Geometry check sheet. Reference: the model listing, model coordinates, mm. A direction names the side the tool comes from. Coordinates: 2 decimals unless noted, no trailing zeros. Order: outer loops, then holes, each group sorted by start corner. A loop starts at its lowest first (then second) coordinate and runs counter-clockwise, first axis right, second up. Notation, with made-up numbers: M -9,-27 L 30,-27 A19 ccw 30,4 Z; hole C 43.5,6 d1. An arc over 180 degrees is marked long. Use CSV: the item, a comma, the result in double quotes. Start each with the question number.
```python
from build123d import *

# Parameters (mm, degrees)
SKETCH_28_R                  = 1
EXTRUDE_4469_DEPTH           = 38
CUT_EXTRUDE_4687_REACH       = 69.476
SKETCH_29_R                  = 1.65
CUT_EXTRUDE_4925_DEPTH       = 51.338851795
FILLET_9_R                   = 3
SKETCH_31_R                  = 1
CUT_EXTRUDE_5310_DEPTH       = 11
SKETCH_32_R                  = 3.5
CUT_EXTRUDE_5556_DEPTH       = 5
HOLE_WIZARD_5601_D           = 3.4
HOLE_WIZARD_5601_CSINK_D     = 6.3
HOLE_WIZARD_5601_CSINK_ANGLE = 90


with BuildPart() as part:
    # Эскиз28 → Extrude 4469 (new body)
    with BuildSketch(Plane.XY):
        Polygon((27, 0), (27, 11), (12, 11), (12, 14), (10, 14), (10, 30), (-20, 30), (-20, 14), (-27, 14), (-27, 11), (-27, 0), align=None)
        with Locations((3, 5.5)):
            Circle(SKETCH_28_R, mode=Mode.SUBTRACT)
        with Locations((-20, 5.5)):
            Circle(SKETCH_28_R, mode=Mode.SUBTRACT)
    extrude(amount=EXTRUDE_4469_DEPTH)

    # Эскиз29 → Cut-Extrude 4687 (cut, up to next)
    with BuildSketch(Plane.ZY.offset(20), mode=Mode.PRIVATE) as cut_extrude_4687_sk1:
        with Locations((6.5, 22)):
            Circle(SKETCH_29_R)
    cut_extrude_4687_tool1 = extrude(cut_extrude_4687_sk1.sketch, amount=-CUT_EXTRUDE_4687_REACH, mode=Mode.PRIVATE) & part.part
    # Эскиз29 → Cut-Extrude 4687 (cut, up to next)
    with BuildSketch(Plane.ZY.offset(20), mode=Mode.PRIVATE) as cut_extrude_4687_sk2:
        with Locations((31.5, 22)):
            Circle(SKETCH_29_R)
    cut_extrude_4687_tool2 = extrude(cut_extrude_4687_sk2.sketch, amount=-CUT_EXTRUDE_4687_REACH, mode=Mode.PRIVATE) & part.part
    add(cut_extrude_4687_tool1.solids().sort_by_distance((-20, 22, 6.5))[0], mode=Mode.SUBTRACT)
    add(cut_extrude_4687_tool2.solids().sort_by_distance((-20, 22, 31.5))[0], mode=Mode.SUBTRACT)

    # Эскиз30 → Cut-Extrude 4925 (cut, through all)
    with BuildSketch(Plane(origin=(0, 11, 0), x_dir=(1, 0, 0), z_dir=(0, 1, 0))):
        with BuildLine():
            Line((23, -13), (16, -13))
            Line((16, -13), (16, -25))
            Line((16, -25), (23, -25))
            ThreePointArc((23, -25), (25.898979486, -27.192752634), (27, -30.656854249))
            Line((27, -30.656854249), (27, -7.343145751))
            ThreePointArc((27, -7.343145751), (25.898979486, -10.807247366), (23, -13))
        make_face()
    extrude(amount=-CUT_EXTRUDE_4925_DEPTH, mode=Mode.SUBTRACT)

    # Скругление9
    # the kernel refuses this fillet: 3 mm, written as the material it takes off along each edge
    with BuildSketch(Plane(origin=(27, 11, 23.156854249), x_dir=(-1, 0, 0), z_dir=(0, 0, 1))) as fillet_9_piece_1:
        with BuildLine():
            CenterArc((FILLET_9_R, FILLET_9_R), FILLET_9_R, 180, 90)
            Line((0, FILLET_9_R), (0, 0))
            Line((0, 0), (FILLET_9_R, 0))
        make_face()
    extrude(amount=22.343145751, mode=Mode.SUBTRACT)
    with BuildSketch(Plane(origin=(27, 11, -7.5), x_dir=(0, -1, 0), z_dir=(0, 0, 1))) as fillet_9_piece_2:
        with BuildLine():
            CenterArc((FILLET_9_R, -FILLET_9_R), FILLET_9_R, 90, 90)
            Line((0, -FILLET_9_R), (0, 0))
            Line((0, 0), (FILLET_9_R, 0))
        make_face()
    extrude(amount=22.343145751, mode=Mode.SUBTRACT)

    # Эскиз31 → Cut-Extrude 5310 (cut)
    with BuildSketch(Plane(origin=(16, 0, 0), x_dir=(0, 0, -1), z_dir=(1, 0, 0))):
        with Locations(Location((-19, 5.5, 0), (0, 0, 90))):
            Circle(SKETCH_31_R)
    extrude(amount=-CUT_EXTRUDE_5310_DEPTH, mode=Mode.SUBTRACT)

    # Эскиз32 → Cut-Extrude 5556 (cut)
    with BuildSketch(Plane(origin=(0, 11, 0), x_dir=(1, 0, 0), z_dir=(0, 1, 0))):
        with Locations(Location((23, -6.5, 0), (0, 0, 180))):
            Circle(SKETCH_32_R)
        with Locations(Location((23, -31.5, 0), (0, 0, 73.398450401))):
            Circle(SKETCH_32_R)
    extrude(amount=-CUT_EXTRUDE_5556_DEPTH, mode=Mode.SUBTRACT)

    # Hole Wizard 5601 (through all)
    with Locations(Plane(origin=(0, 6, 0), x_dir=(1, 0, 0), z_dir=(0, 1, 0))):
        with Locations((23, -6.5), (23, -31.5)):
            CounterSinkHole(HOLE_WIZARD_5601_D / 2, HOLE_WIZARD_5601_CSINK_D / 2, counter_sink_angle=HOLE_WIZARD_5601_CSINK_ANGLE)


solid = part.part
```
1) Section check C-C on z = 6.5. Record the boundary of the cut face in (x, y), then the cut area to 3 significant figures.
2) Section check B-B on y = 22. Record the boundary of the cut face in (x, z).
3) Draft check along Y on faces 6 (the face through (11, 14, 19)), 7 (the face through (2.87, 6.49, 18.73)), 8 (the face through (21.43, 2.24, 7.15)). Enter one of: +Y half, -Y half, draft (parallel to the pull), parting line (faces both ways), or undercut.
4) Gauge pin test, flat ends, axial feed: P1, Ø3, axis at y = 13.5, z = 30.5, coming from the +X side; P2, Ø17.5, axis at y = 23, z = 11, coming from the -X side; P3, Ø3, axis at x = 12, z = 12, coming from the +Y side; P4, Ø12, axis at x = 18, y = 12, coming from the -Z side. Record the tip position at first contact, or that the pin passes through.
5) Section check D-D on z = 19. Record the boundary of the cut face in (x, y), then the cut area to 3 significant figures.
6) Set-up check for faces 1 (the face through (19.767, 8.535, 5.159)), 2 (the face through (-20, 22, 19)), 3 (the face through (16, 7, 19)), 4 (the face through (-20.737, 6.176, 18.734)), 5 (the face through (12, 12, 19)): record each of +Z, -Z, +X, -X, +Y, -Y from which the full face is reachable in a straight line by a thin tool's end or side.
7) Section check A-A on x = 3. Record the boundary of the cut face in (y, z), then the cut area to 3 significant figures.
8) Material ranges on line 1 along Z through (x, y) = (23, 9.35); line 2 along Z through (x, y) = (23, 2); line 3 along X through (y, z) = (8.2, 31.5), recorded low to high.
Results are:
1,outline,"M -27,0 L 21.3,0 L 21.3,4.55 L 19.85,6 L 19.5,6 L 19.5,11 L 12,11 L 12,14 L 10,14 L 10,20.35 L -20,20.35 L -20,14 L -27,14 Z; M -20,23.65 L 10,23.65 L 10,30 L -20,30 Z; M 24.7,0 L 27,0 L 27,8 A3 ccw 26.5,9.66 L 26.5,6 L 26.15,6 L 24.7,4.55 Z; hole C -20,5.5 d2; hole C 3,5.5 d2"
1,area,"1,030 mm²"
2,outline,"M -20,0 L 10,0 L 10,4.85 L -20,4.85 Z; M -20,8.15 L 10,8.15 L 10,29.85 L -20,29.85 Z; M -20,33.15 L 10,33.15 L 10,38 L -20,38 Z"
3,face 6,"+Y half"
3,face 7,"undercut"
3,face 8,"draft"
4,P1,"stops at x = 12"
4,P2,"stops at x = -20"
4,P3,"stops at y = 14"
4,P4,"stops at z = 0"
5,outline,"M -27,0 L 16,0 L 16,4.5 L 5,4.5 L 5,6.5 L 16,6.5 L 16,11 L 12,11 L 12,14 L 10,14 L 10,30 L -20,30 L -20,14 L -27,14 Z; hole C -20,5.5 d2; hole C 3,5.5 d2"
5,area,"1,040 mm²"
6,face 1,"+Y"
6,face 2,"+Z, -Z, -X, +Y"
6,face 3,"+X, +Y, -Y"
6,face 4,"+Z, -Z"
6,face 5,"+Z, -Z, +X, +Y"
7,outline,"M 0,0 L 4.5,0 L 4.5,38 L 0,38 Z; M 6.5,0 L 30,0 L 30,38 L 6.5,38 Z; hole C 22,6.5 d3.3; hole C 22,31.5 d3.3"
7,area,"1,050 mm²"
8,line 1,"z = 0 to 3, 10 to 13, 25 to 28, 35 to 38"
8,line 2,"z = 0 to 4.8, 8.2 to 13, 25 to 29.8, 33.2 to 38"
8,line 3,"x = -27 to 19.5, 26.5 to 26.99"
